```python
from build123d import *

# Parameters (mm, degrees)
F0_W     = 10
F0_H     = 6
F1_DEPTH = 5
F2_R     = 4.9247083424
F3_DEPTH = 20
F4_R     = 4.9247083424
F5_DEPTH = 4


with BuildPart() as f1:
    # F0 (on Top) → F1 (new body, symmetric)
    with BuildSketch(Plane.XY):
        Polygon((29.5, -29.5), (-29.5, -29.5), (-39.5, -29.5), (-39.5, -38.1432852078), (39.5, -38.1432852078), (39.5, 38.1432852078), (-39.5, 38.1432852078), (-39.5, 23.5), (-29.5, 23.5), (-29.5, 29.5), (29.5, 29.5), align=None)
        with Locations((-34.5, -26.5)):
            Rectangle(F0_W, F0_H)
    extrude(amount=F1_DEPTH, both=True)

    # F2 (on face) → F3 (join)
    with BuildSketch(Plane(origin=(0, 38.1432852078, 0), x_dir=(-1, 0, 0), z_dir=(0, 1, 0))):
        Circle(F2_R)
    extrude(amount=F3_DEPTH)

    # F4 (on face) → F5 (join)
    with BuildSketch(Plane(origin=(0, 58.1432852078, 0), x_dir=(-1, 0, 0), z_dir=(0, 1, 0))):
        with BuildLine():
            ThreePointArc((-8.6772361623, 4.9704700566), (-2.5717346653, -9.6636525606), (10, 0))
            ThreePointArc((10, 0), (9.6636525606, 2.5717346653), (8.6772361623, 4.9704700566))
            Line((8.6772361623, 4.9704700566), (-8.6772361623, 4.9704700566))
        make_face()
        Circle(F4_R, mode=Mode.SUBTRACT)
        Circle(F4_R)
    extrude(amount=F5_DEPTH)


solid = f1.part
```
The model under review builds one solid part; all positions refer to its coordinate system, in mm. A direction names the side the tool comes from. Round coordinates to 2 decimals unless told otherwise and drop trailing zeros. Write each loop counter-clockwise with the first axis right and the second up, starting at its lowest first coordinate (ties: lowest second). Pieces come first, ordered by that corner, then holes. Notation, with made-up numbers: (85.5, 9.25) - (122.5, 9.25) arc R18 cw to (122.5, 26.25) - close; hole circle Ø5 at (58, 68.25). An arc over 180 degrees is marked (long way). Use one line per item in the form item = value.
Q1. Consider section A-A (x = 0). State the section outline as (y, z) points, and give its area (3 significant figures).
Answer key:
outline = (-38.14, -5) - (-29.5, -5) - (-29.5, 5) - (-38.14, 5) - close; (29.5, -5) - (38.14, -5) - (38.14, -4.92) - (58.14, -4.92) - (58.14, -10) - (62.14, -10) - (62.14, 4.97) - (58.14, 4.97) - (58.14, 4.92) - (38.14, 4.92) - (38.14, 5) - (29.5, 5) - close
area = 430 mm2
Q2. Draft analysis for pull direction Y (two halves, no side actions). For faces 1 (the flat face through (0, 29.5, 0)), 2 (the flat face through (-1, -38.143, 0)), 3 (the flat face through (0, 62.143, -1)), 4 (the flat face through (39.5, -1, 0)), state which applies: +Y half, -Y half, draft (parallel to the pull), parting line (faces both ways), or undercut.
Answer key:
face_1 = undercut
face_2 = -Y half
face_3 = +Y half
face_4 = draft
Q3. Consider section B-B (y = 16.5). State the section outline as (x, z) points.
Answer key:
outline = (29.5, -5) - (39.5, -5) - (39.5, 5) - (29.5, 5) - close
Q4. For line 1 (Y direction, x = 5, z = 2.5); line 2 (Y direction, x = -30, z = -1); line 3 (Y direction, x = -28, z = -3), list the stretches that pass through material, from the lowest coordinate up. Write a range as [from, to].
Answer key:
line_1 = [-38.14, -29.5], [29.5, 38.14], [58.14, 62.14]
line_2 = [-38.14, -23.5], [23.5, 38.14]
line_3 = [-38.14, -29.5], [29.5, 38.14]
Q5. Insertion check: pin 1 Ø3 at (x, z) = (-10.5, -7) entering from +Y; pin 2 Ø3 at (x, y) = (-2, 59.5) entering from +Z; pin 3 Ø8 at (y, z) = (-5.5, -2.5) entering from -X; pin 4 Ø8 at (x, z) = (-35.5, -1.5) entering from +Y. Each pin has a flat end and moves straight along its axis. Give the tip position at first contact, or say it passes through.
Answer key:
pin_1 = through
pin_2 = 4.97
pin_3 = 29.5
pin_4 = 38.14
Q6. Consider section D-D (z = -8). State the section outline as (x, y) points, and give its area (3 significant figures).
Answer key:
outline = (-6, 58.14) - (6, 58.14) - (6, 62.14) - (-6, 62.14) - close
area = 48.0 mm2
Q7. Consider section C-C (x = 13.5). State the section outline as (y, z) points, and give its area (3 significant figures).
Answer key:
outline = (-38.14, -5) - (-29.5, -5) - (-29.5, 5) - (-38.14, 5) - close; (29.5, -5) - (38.14, -5) - (38.14, 5) - (29.5, 5) - close
area = 173 mm2
Q8. Tool access review of faces 5 (the flat face through (-35, -23.5, 0)), 6 (the flat face through (-29.5, 26, 0)), 7 (the cylindrical face through (-4.697, 48.003, 1.479)), 8 (the flat face through (32, 0, -5)): name each direction out of +Z, -Z, +X, -X, +Y, -Y from which nothing blocks a thin tool from reaching the whole face with its end or side.
Answer key:
face_5 = +Z, -Z, -X
face_6 = +Z, -Z
face_7 = none
face_8 = -Z, +X, -X, -Y
